Geometry: final body of the model. Coordinates: model frame, mm. A direction names the side the tool comes from. Round coordinates to 2 decimals unless told otherwise and drop trailing zeros. Loops run counter-clockwise (first coordinate to the right, second up) from the corner with the lowest first, then second, coordinate; pieces in that order, holes last. Notation, with made-up numbers: (25, 44) - (45, 44) arc R26 cw to (45, 83) - close; hole circle Ø4 at (-25, 58). An arc over 180 degrees is marked (long way). Answer as a JSON object with one key per item and string values. Group by question number.
Item 1: Line query: line 1 (Y direction, x = 17, z = 8.5); line 2 (Y direction, x = 31.5, z = 7.75); line 3 (Y direction, x = -2.5, z = 6). Output: solid intervals per line, ascending.
Item 2: Reachability of faces 5 (the face through (6.17, 58.8, 11.51)), 6 (the face through (-4.8, 90.5, 6.1)) from +Z, -Z, +X, -X, +Y, -Y: full face, straight path, thin tool, end or side. Return the list, or none.
Item 3: First-contact query: pin 1 (5 mm diameter, centred on x = 42, z = 3.5, fed in from +Y); pin 2 (3 mm diameter, centred on x = -6, z = 9, fed in from -Y); pin 3 (2 mm diameter, centred on y = 60.5, z = 9, fed in from -X). Flat tips, straight axial feed; report the tip coordinate or a pass-through.
Item 4: Section D-D (x = 6.5). Return the cut outline in (y, z).
Item 5: Draft query along Y for faces 1 (the face through (-5, 88, 6)), 2 (the face through (-8.244, 96.514, 6.084)), 3 (the face through (0, 45, 6)), 4 (the face through (49, 12, 6)). Return one class per face: released by +Y, released by -Y, zero draft, split by the parting line, or undercut.
Item 6: Section A-A (x = 69.5). Return the cut outline in (y, z), plus the area to 3 significant figures.
Item 7: Section B-B (z = 3). Count the separate pieces of the cut face and the enclosed holes in it, plus the area to 3 significant figures.
```python
from build123d import *

# Parameters (mm, degrees)
F0_R         = 3.5
F1_DEPTH     = 12
F3_DEPTH     = 25
F4_R         = 5
F5_W         = 12
F5_H         = 12
F6_DEPTH     = 10
F8_T1_DEPTH  = 86.6740446023
F8_T3_DEPTH  = 16.6151120325
F8_T5_DEPTH  = 82.571682988
F8_T7_DEPTH  = 63.5360023124
F8_T10_ANGLE = 180
F8_T12_ANGLE = 83.5169263071
F8_T14_ANGLE = 180
F8_T16_ANGLE = 83.5169263071
F9_DEPTH     = 25


# Not quite as in the source:
# - a fillet or chamfer that OpenCascade refuses, or shapes differently, is made with other operations: its cross-section is extruded or revolved along the edge and cut away or added


with BuildPart() as f1:
    # F0 (on Top) → F1 (new body)
    with BuildSketch(Plane.XY):
        with BuildLine():
            Line((12, 100), (0, 100))
            Line((0, 100), (0, 0))
            Line((0, 0), (80, 0))
            ThreePointArc((80, 0), (86, 6), (80, 12))
            Line((80, 12), (12, 12))
            Line((12, 12), (12, 100))
        make_face()
        with Locations((6.5, 6)):
            Circle(F0_R, mode=Mode.SUBTRACT)
        with Locations((17, 6)):
            Circle(F0_R, mode=Mode.SUBTRACT)
        with Locations((27.5, 6)):
            Circle(F0_R, mode=Mode.SUBTRACT)
        with Locations((38, 6)):
            Circle(F0_R, mode=Mode.SUBTRACT)
        with Locations((48.5, 6)):
            Circle(F0_R, mode=Mode.SUBTRACT)
        with Locations((59, 6)):
            Circle(F0_R, mode=Mode.SUBTRACT)
        with Locations((69.5, 6)):
            Circle(F0_R, mode=Mode.SUBTRACT)
        with Locations((80, 6)):
            Circle(F0_R, mode=Mode.SUBTRACT)
    extrude(amount=F1_DEPTH)

    # F2 (on face) → F3 (cut)
    with BuildSketch(Plane.XY.offset(12)):
        Polygon((2, 100), (12, 12), (12, 100), align=None)
    extrude(amount=-F3_DEPTH, mode=Mode.SUBTRACT)

    # F4
    f4_edges = [f1.edges().sort_by_distance(p)[0] for p in [
        (12, 12, 6),
    ]]
    fillet(f4_edges, radius=F4_R)

    # F5 (on face) → F6 (join)
    with BuildSketch(Plane(origin=(0, 0, 0), x_dir=(0, -1, 0), z_dir=(-1, 0, 0))):
        with Locations((-94, 6)):
            Rectangle(F5_W, F5_H)
    extrude(amount=F6_DEPTH)

    # F8: chamfer of 1 on 11 edges, made by hand

    # F8_s2 → F8_t1 (cut)
    with BuildSketch(Plane(origin=(-11.4836366644, 101.0560026464, 0), x_dir=(0, 0, 1), z_dir=(0.112909688, -0.9936052548, 0))):
        Polygon((12, -12.278179314), (11, -13.278179314), (12, -13.278179314), align=None)
        Polygon((0, -12.278179314), (1, -13.278179314), (0, -13.278179314), align=None)
    extrude(amount=F8_T1_DEPTH, mode=Mode.SUBTRACT)

    # F8_s4 → F8_t3 (cut)
    with BuildSketch(Plane.XY.offset(-2.3075560163)):
        Polygon((1.1072004625, 100), (2.1008057173, 99.112909688), (2, 100), align=None)
    extrude(amount=F8_T3_DEPTH, mode=Mode.SUBTRACT)

    # F8_s6 → F8_t5 (cut)
    with BuildSketch(Plane.YZ.offset(-2.571682988)):
        Polygon((1, 0), (0, 1), (0, 0), align=None)
        Polygon((1, 12), (0, 11), (0, 12), align=None)
    extrude(amount=F8_T5_DEPTH, mode=Mode.SUBTRACT)

    # F8_s8 → F8_t7 (cut)
    with BuildSketch(Plane.YZ.offset(16.4639976876)):
        Polygon((11, 0), (12, 1), (12, 0), align=None)
        Polygon((11, 12), (12, 11), (12, 12), align=None)
    extrude(amount=F8_T7_DEPTH, mode=Mode.SUBTRACT)

    # F8_s9 → F8_t10 (revolve, cut)
    with BuildSketch(Plane.YZ.offset(80)):
        Polygon((1, 0), (0, 1), (0, 0), align=None)
    revolve(axis=Axis((80, 6, 0), (0, 0, 1)), revolution_arc=F8_T10_ANGLE, mode=Mode.SUBTRACT)

    # F8_s11 → F8_t12 (revolve, cut)
    with BuildSketch(Plane(origin=(-1.6972973268, 14.9362164756, 0), x_dir=(0, 0, 1), z_dir=(-0.112909688, 0.9936052548, 0))):
        Polygon((0, 12.278179314), (1, 13.278179314), (0, 13.278179314), align=None)
    revolve(axis=Axis((16.4639976876, 17, 0), (0, 0, 1)), revolution_arc=F8_T12_ANGLE, mode=Mode.SUBTRACT)

    # F8_s13 → F8_t14 (revolve, cut)
    with BuildSketch(Plane.YZ.offset(80)):
        Polygon((1, 12), (0, 11), (0, 12), align=None)
    revolve(axis=Axis((80, 6, 12), (0, 0, 1)), revolution_arc=F8_T14_ANGLE, mode=Mode.SUBTRACT)

    # F8_s15 → F8_t16 (revolve, cut)
    with BuildSketch(Plane(origin=(-1.6972973268, 14.9362164756, 0), x_dir=(0, 0, 1), z_dir=(-0.112909688, 0.9936052548, 0))):
        Polygon((12, 12.278179314), (11, 13.278179314), (12, 13.278179314), align=None)
    revolve(axis=Axis((16.4639976876, 17, 12), (0, 0, 1)), revolution_arc=F8_T16_ANGLE, mode=Mode.SUBTRACT)

    # F7 (on face) → F9 (cut)
    with BuildSketch(Plane.XY.offset(12)):
        Polygon((150.627374606, 89.5), (150.627374606, 97.5), (143.6991713757, 101.5), (136.7709681454, 97.5), (136.7709681454, 89.5), (143.6991713757, 85.5), align=None)
        Polygon((-6.536, 89.5), (-3.0718983849, 91.5), (-3.0718983849, 95.5), (-6.536, 97.5), (-10.0001016151, 95.5), (-10.0001016151, 91.5), align=None)
    extrude(amount=-F9_DEPTH, mode=Mode.SUBTRACT)


solid = f1.part
```
Values:
{
 "1": {"line 1": "y = 0 to 2.5, 9.5 to 12", "line 2": "y = 0 to 12", "line 3": "y = 88 to 100"},
 "2": {"face 5": "+Z, +X, +Y", "face 6": "+Z, -Z"},
 "3": {"pin 1": "stops at y = 12", "pin 2": "stops at y = 88", "pin 3": "stops at x = 0"},
 "4": {"outline": "(0, 1) - (1, 0) - (2.5, 0) - (2.5, 12) - (1, 12) - (0, 11) - close; (9.5, 0) - (51.54, 0) - (60.4, 1) - (60.4, 11) - (51.54, 12) - (9.5, 12) - close"},
 "5": {"face 1": "released by -Y", "face 2": "undercut", "face 3": "zero draft", "face 4": "released by +Y"},
 "6": {"outline": "(0, 1) - (1, 0) - (2.5, 0) - (2.5, 12) - (1, 12) - (0, 11) - close; (9.5, 0) - (11, 0) - (12, 1) - (12, 11) - (11, 12) - (9.5, 12) - close", "area": "58.0 mm^2"},
 "7": {"separate pieces": "1", "enclosed holes": "8", "area": "1,410 mm^2"}
}
